Work out the finished part from the listing and answer in its coordinate system (mm). A direction names the side the tool comes from. Coordinates: 2 decimals unless noted, no trailing zeros. Write each loop counter-clockwise with the first axis right and the second up, starting at its lowest first coordinate (ties: lowest second). Pieces come first, ordered by that corner, then holes. Notation, with made-up numbers: (-1.75, -36.5) - (17.25, -36.5) arc R20 cw to (17.25, -8.5) - close; hole circle Ø5 at (89.25, 37). An arc over 180 degrees is marked (long way). Use one line per item in the form item = value. Start each with the question number.
Item 1: A cutting plane is placed at B-B (x = -64). Write down the section's boundary in (y, z).
Item 2: A cutting plane is placed at A-A (y = 65). Write down the section's boundary in (x, z).
Item 3: Determine the mould class of faces 3 (the flat face through (-3, 15, 143)), 4 (the flat face through (-59.86, 65.7, 280.14)), 5 (the flat face through (-1, 42, 0)) for opening direction Z: released by +Z, released by -Z, zero draft, split by the parting line, or undercut.
Item 4: Given pin 1 (5 mm diameter, centred on x = 6.5, z = 202, fed in from +Y), flat-ended and moving along its own axis, determine where the tip first touches the part or whether it passes through.
Item 5: For faces 1 (the flat face through (-1, 74, 20)), 2 (the flat face through (-59.86, 65.7, 10.14)), determine the directions among +Z, -Z, +X, -X, +Y, -Y from which every point of the face is accessible in a straight line to the end or side of a thin tool.
Item 6: A cutting plane is placed at D-D (z = 249). Write down the section's boundary in (x, y), then the cut area to 3 significant figures.
Item 7: Consider probe 1 along Z at (x, y) = (-19.5, 146.5); probe 2 along Y at (x, z) = (-11.5, 46.5). Determine where each line is inside the solid, lowest interval first.
Item 8: A cutting plane is placed at C-C (y = 36). Write down the section's boundary in (x, z).
from build123d import *

# Parameters (mm, degrees)
SKETCH1_W           = 400
SKETCH1_H           = 30
BOSS_EXTRUDE1_DEPTH = 290
BOSS_EXTRUDE2_DEPTH = 20
SKETCH4_R           = 25
CUT_EXTRUDE1_DEPTH  = 20
BOSS_EXTRUDE3_START = -20
SKETCH5_R           = 25
BOSS_EXTRUDE3_DEPTH = 20


with BuildPart() as part:
    # Sketch1 → Boss-Extrude1 (new body)
    with BuildSketch(Plane.XY):
        Rectangle(SKETCH1_W, SKETCH1_H)
    extrude(amount=BOSS_EXTRUDE1_DEPTH)

    # Sketch2 → Boss-Extrude2 (add)
    with BuildSketch(Plane.XY.offset(290)):
        with BuildLine():
            Line((0, 165), (0, 115))
            Line((0, 115), (50, 115))
            ThreePointArc((50, 115), (32.360636061, 147.360636061), (0, 165))
        make_face()
        with BuildLine():
            Line((-50, 115), (0, 115))
            Line((0, 115), (0, 165))
            ThreePointArc((0, 165), (-32.360636061, 147.360636061), (-50, 115))
        make_face()
        Polygon((-70, 15), (0, 15), (0, 115), (-50, 115), align=None)
        Polygon((0, 115), (0, 15), (70, 15), (50, 115), align=None)
    extrude(amount=-BOSS_EXTRUDE2_DEPTH)

    # Sketch4 → Cut-Extrude1 (cut)
    with BuildSketch(Plane.XY.offset(290)):
        with Locations((0, 116.092070287)):
            Circle(SKETCH4_R)
    extrude(amount=-CUT_EXTRUDE1_DEPTH, mode=Mode.SUBTRACT)

    # Sketch5 → Boss-Extrude3 (add)
    with BuildSketch(Plane(origin=(0, 0, 0), x_dir=(-1, 0, 0), z_dir=(0, 0, -1)).offset(BOSS_EXTRUDE3_START)):
        with BuildLine():
            Line((-70, 15), (-50, 115))
            ThreePointArc((-50, 115), (-32.360636061, 147.360636061), (0, 165))
            ThreePointArc((0, 165), (32.360636061, 147.360636061), (50, 115))
            Line((50, 115), (70, 15))
            Line((70, 15), (-70, 15))
        make_face()
        with Locations(Location((0, 116.092070287, 0), (0, 0, 180))):
            Circle(SKETCH5_R, mode=Mode.SUBTRACT)
    extrude(amount=BOSS_EXTRUDE3_DEPTH)


solid = part.part
Answer:
q1.outline = (-15, 0) - (45, 0) - (45, 20) - (15, 20) - (15, 270) - (45, 270) - (45, 290) - (-15, 290) - close
q2.outline = (-60, 0) - (60, 0) - (60, 20) - (-60, 20) - close; (-60, 270) - (60, 270) - (60, 290) - (-60, 290) - close
q3.face_3 = undercut
q3.face_4 = zero draft
q3.face_5 = released by -Z
q4.pin_1 = 15
q5.face_1 = +X, -X, +Y
q5.face_2 = +Z, -Z, -X, +Y
q6.outline = (-200, -15) - (200, -15) - (200, 15) - (-200, 15) - close
q6.area = 12,000 mm²
q7.probe_1 = 0 to 20, 270 to 290
q7.probe_2 = -15 to 15
q8.outline = (-65.8, 0) - (65.8, 0) - (65.8, 20) - (-65.8, 20) - close; (-65.8, 270) - (65.8, 270) - (65.8, 290) - (-65.8, 290) - close
